Design review of the part shown in the three views and the two pictorial views. Dimensions are in mm from the part's minimum x, y and z. Coordinates: 2 decimals unless noted, no trailing zeros. Write each loop counter-clockwise with the first axis right and the second up, starting at its lowest first coordinate (ties: lowest second). Pieces come first, ordered by that corner, then holes. Notation, with made-up numbers: (41, -2) -> (46, -2) arc R15 ccw to (46, 3) -> close; hole circle Ø4 at (52.5, 82.5). An arc over 180 degrees is marked (long way). Write each question's results on one line, items separated by ' | '.
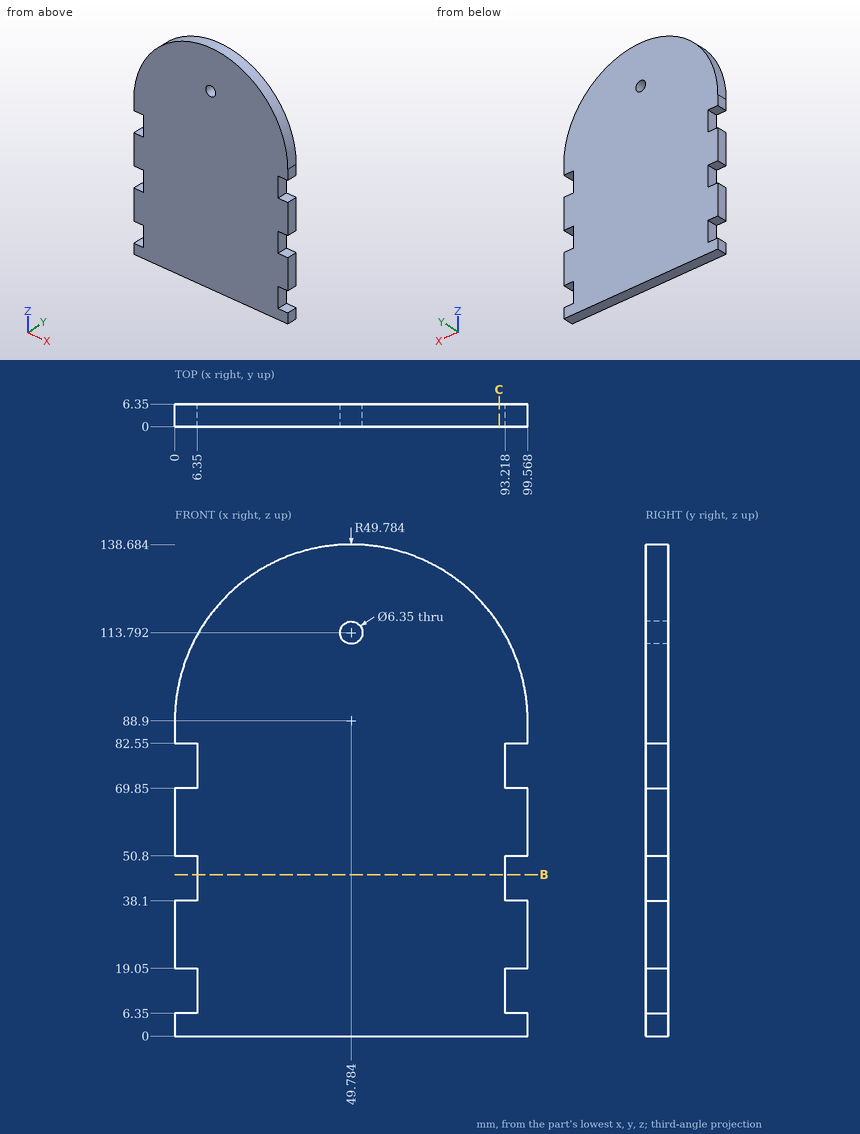
Q1. Add section B-B (z = 45.5). Write out the cut boundary in (x, y).
Solution:
outline: (6.35, 0) -> (93.22, 0) -> (93.22, 6.35) -> (6.35, 6.35) -> close
Q2. Clearance check with flat-ended pins moving along their axes: P1, Ø2, axis at x = 37, y = 4, coming from the +Z side; P2, Ø1.9, axis at y = 2, z = 45, coming from the -X side; P3, Ø1.9, axis at x = 96.5, y = 3.5, coming from the +Z side. State where each tip first meets the part, or that it passes through.
Solution:
P1: z = 137.27 | P2: x = 6.35 | P3: z = 108.49
Q3. Add section C-C (x = 91.5). Write out the cut boundary in (y, z).
Solution:
outline: (0, 0) -> (6.35, 0) -> (6.35, 116.07) -> (0, 116.07) -> close
Q4. For line 1 (X direction, y = 1.5, z = 8.5); line 2 (Z direction, x = 48, y = 5.75); line 3 (Z direction, x = 41, y = 4.5), list the stretches that pass through material, from the lowest coordinate up. Write a range as from..to.
Solution:
line 1: 6.35..93.22 | line 2: 0..111.17, 116.42..138.65 | line 3: 0..137.9
